Drawing for the job (mm, zero at the part's lowest x, y, z). A direction names the side the tool comes from. Coordinates: 2 decimals unless noted, no trailing zeros. Write each loop counter-clockwise with the first axis right and the second up, starting at its lowest first coordinate (ties: lowest second). Pieces come first, ordered by that corner, then holes. Notation, with made-up numbers: M 29.5,4.25 L 41.5,4.25 A14 cw 41.5,20.25 Z; hole C -15.5,47 d2. An arc over 180 degrees is marked long. Put each result on its own line as item: value. Start each with the question number.
Q1. Pull direction Y, two halves, no side cores. Call the marked faces 3 and 4: pulls with the +Y half, pulls with the -Y half, needs draft (parallel to the pull), parting line crosses it, or undercut.
Q2. Drill centre lines: line 1 along Y through (x, z) = (2.25, 3.5); line 2 along Z through (x, y) = (21.5, 10); line 3 along X through (y, z) = (1.25, 2.25). Where is each one in solid material? Low to high.
Q3. Cut at D-D (z = 7.75). Write the cut outline in (x, y).
Q4. Which spindle directions (+Z, -Z, +X, -X, +Y, -Y) get a long thin tool onto all of the face, cutting with end or side? Do the marked faces 1 and 2. Say none if no direction does.
Q5. Cut at C-C (x = 9.5). Write the cut outline in (y, z).
Q6. Cut at A-A (y = 5.5). Write the cut outline in (x, z).
Q7. Cut at B-B (z = 5.5). Write the cut outline in (x, y), then the cut area to 3 significant figures.
Q8. Drop a flat-ended pin along its axis: pin 1 (1.9 mm diameter, centred on x = 12, y = 4.5, fed in from +Z). Give the stop position or say it passes through.
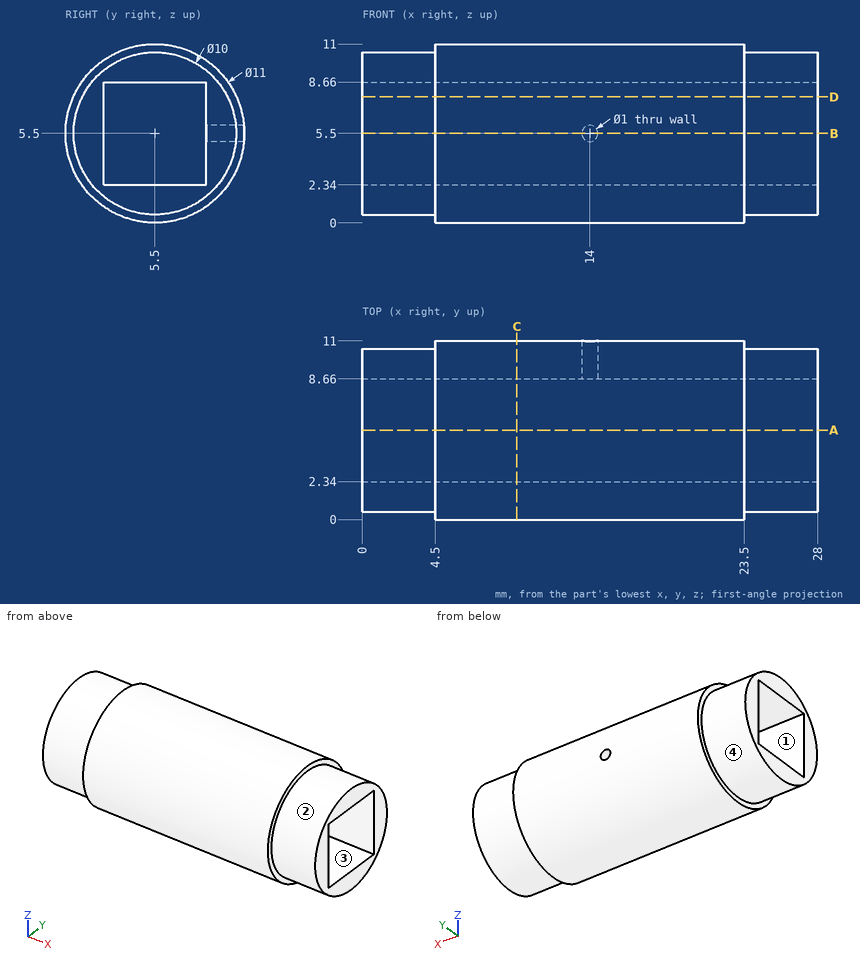
Computed values:
1. face 3: undercut
1. face 4: parting line crosses it
2. line 1: 0.92 to 2.34, 8.66 to 10.08
2. line 2: 2.34 to 8.66
2. line 3: 4.5 to 23.5
3. outline: M 0,1.03 L 4.5,1.03 L 4.5,0.48 L 23.5,0.48 L 23.5,1.03 L 28,1.03 L 28,2.34 L 0,2.34 Z; M 0,8.66 L 28,8.66 L 28,9.97 L 23.5,9.97 L 23.5,10.52 L 4.5,10.52 L 4.5,9.97 L 0,9.97 Z
4. face 1: +X, -X
4. face 2: +X
5. outline: C 5.5,5.5 d11; hole M 2.34,2.34 L 8.66,2.34 L 8.66,8.66 L 2.34,8.66 Z
6. outline: M 0,0.5 L 4.5,0.5 L 4.5,0 L 23.5,0 L 23.5,0.5 L 28,0.5 L 28,2.34 L 0,2.34 Z; M 0,8.66 L 28,8.66 L 28,10.5 L 23.5,10.5 L 23.5,11 L 4.5,11 L 4.5,10.5 L 0,10.5 Z
7. outline: M 0,0.5 L 4.5,0.5 L 4.5,0 L 23.5,0 L 23.5,0.5 L 28,0.5 L 28,2.34 L 0,2.34 Z; M 0,8.66 L 13.5,8.66 L 13.5,11 L 4.5,11 L 4.5,10.5 L 0,10.5 Z; M 14.5,8.66 L 28,8.66 L 28,10.5 L 23.5,10.5 L 23.5,11 L 14.5,11 Z
7. area: 120 mm2
8. pin 1: z = 11
